Input: part model. Units: mm. Frame: model coordinates. Face numbers are marked on the shaded views. A direction names the side the tool comes from. Coordinates: 2 decimals unless noted, no trailing zeros. Write each loop counter-clockwise with the first axis right and the second up, starting at its lowest first coordinate (ties: lowest second). Pieces come first, ordered by that corner, then holes. Notation, with made-up numbers: (-4.5, 85.25) - (24.5, 85.25) arc R7 cw to (24.5, 98.25) - close; hole circle Ø6 at (87.5, 46). An arc over 180 degrees is marked (long way). Put each result on its own line as item: value. Start each with the question number.
1. Cut plane C-C, the plane y = 6.25. Return loops of the section in (x, z), and give its area (3 significant figures).
2. Cut plane D-D, the plane y = 2. Return loops of the section in (x, z).
3. Line query: line 1 (Z direction, x = 4, y = 5.5); line 2 (X direction, y = -0.2, z = -11.75); line 3 (Z direction, x = 18, y = -2). Output: solid intervals per line, ascending.
4. Pull-direction query (Z, two-part tool) for the marked faces 3, 4 and 5; classes: released by +Z, released by -Z, zero draft, split by the parting line, or undercut.
5. Cut plane B-B, the plane z = -11.75. Return loops of the section in (x, y), and give its area (3 significant figures).
6. Access query for the marked faces 1 and 2. Directions: +Z, -Z, +X, -X, +Y, -Y. A direction counts if a zero-diameter tool reaches every point of the face in a straight line with its end or side. Return the directions, or none.
7. Pin query (flat end, axial travel): pin 1 (11.5 mm diameter, centred on x = 17.5, z = 11.75, fed in from +Y); pin 2 (2.5 mm diameter, centred on y = -3.5, z = 15, fed in from -X); pin 3 (14.5 mm diameter, centred on x = 13, z = 1.5, fed in from +Y). Return the tip coordinate at first contact, or that it passes through.
8. Cut plane A-A, the plane x = 17.5. Return loops of the section in (y, z), and give its area (4 significant figures).
from build123d import *

# Parameters (mm, degrees)
EXTRUDE_1_DEPTH          = 22
PATTERN_LINEAR_1_COUNT   = 2
PATTERN_LINEAR_1_PITCH   = 23.5
CUT_EXTRUDE_1_DEPTH      = 38.269290307
CUT_EXTRUDE_1_DEPTH_BACK = 38.269290307
SKETCH_4_W               = 16.100903004
SKETCH_4_H               = 10.25
SKETCH_5_R               = 2.5
CUT_EXTRUDE_2_DEPTH      = 54.301031885


with BuildPart() as part:
    # 草图1 → 凸台-拉伸1 (new, symmetric)
    with BuildSketch(Plane.XY):
        with BuildLine():
            Line((29, -5.5), (29, -8))
            Line((29, -8), (1, -8))
            Line((1, -8), (-1.370141735, -7.373785434))
            ThreePointArc((-1.370141735, -7.373785434), (-4.794472702, 5.767411162), (7.5, 0))
            Line((7.5, 0), (25.406366901, 0))
            ThreePointArc((25.406366901, 0), (25.916831332, -0.140101131), (26.284262474, -0.521147869))
            Line((26.284262474, -0.521147869), (29, -5.5))
        make_face()
    extrude(amount=EXTRUDE_1_DEPTH, both=True)

    # 草图3 → 切除-旋转1 (revolve, cut)
    with BuildSketch(Plane.XY.offset(11.75), mode=Mode.PRIVATE) as cut_revolve_1_sk:
        Polygon((24, 0), (17.5, 0), (17.5, -8), (20.75, -8), (20.75, -4), (24, -1), align=None)
    cut_revolve_1 = revolve(cut_revolve_1_sk.sketch.rotate(Axis((17.5, -8, 11.75), (0, 1, 0)), 90), axis=Axis((17.5, -8, 11.75), (0, 1, 0)), mode=Mode.SUBTRACT)

    # 阵列(线性)1: 切除-旋转1 ×2
    with Locations(*[(0, 0, -i * PATTERN_LINEAR_1_PITCH) for i in range(1, PATTERN_LINEAR_1_COUNT)]):
        add(cut_revolve_1, mode=Mode.SUBTRACT)

    # 草图4 → 切除-拉伸1 (cut, two sides: drawn at the far end of the back side and taken through both)
    with BuildSketch(Plane(origin=(0, 0, 0), x_dir=(1, 0, 0), z_dir=(0, 1, 0)).offset(-CUT_EXTRUDE_1_DEPTH_BACK)):
        with Locations((-0.04685673, -16.875)):
            Rectangle(SKETCH_4_W, SKETCH_4_H)
        with Locations((-0.04685673, 5.625)):
            Rectangle(SKETCH_4_W, SKETCH_4_H)
    extrude(amount=CUT_EXTRUDE_1_DEPTH + CUT_EXTRUDE_1_DEPTH_BACK, mode=Mode.SUBTRACT)

    # 草图5 → 切除-拉伸2 (cut, through all)
    with BuildSketch(Plane(origin=(0, 0, -22), x_dir=(-1, 0, 0), z_dir=(0, 0, -1))):
        Circle(SKETCH_5_R)
    extrude(amount=-CUT_EXTRUDE_2_DEPTH, mode=Mode.SUBTRACT)


solid = part.part
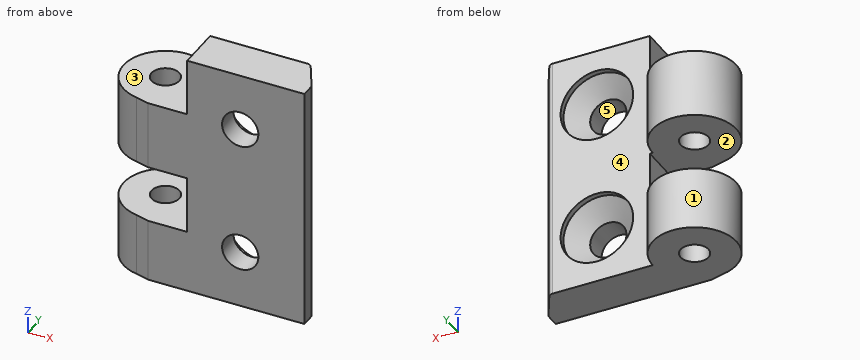
Report:
1. outline: (-4.15, -22) - (4.15, -22) - (4.15, -10.75) - (-4.15, -10.75) - close; (-4.15, -0.5) - (4.15, -0.5) - (4.15, 11.75) - (-4.15, 11.75) - close
1. area: 195 mm^2
2. outline: (-7.23, -22) - (-1.5, -22) - (-1.5, -10.75) - (-7.23, -10.75) - close; (-7.23, -0.5) - (-1.5, -0.5) - (-1.5, 11.75) - (-7.23, 11.75) - close; (1.5, -22) - (7.23, -22) - (7.23, -10.75) - (1.5, -10.75) - close; (1.5, -0.5) - (7.23, -0.5) - (7.23, 11.75) - (1.5, 11.75) - close
3. line 1: z = -22 to -10.75, -0.5 to 11.75
3. line 2: x = -7.5 to -2.49, 2.49 to 11, 24 to 26.01
3. line 3: z = -22 to -17.14, -6.36 to 6.36, 17.14 to 22
4. face 3: released by +Z
4. face 4: zero draft
4. face 5: undercut
5. outline: (-1.37, -7.37) - (1, -8) - (14.25, -8) - (14.25, -4) - (11, -1) - (11, 0) - (7.5, 0) arc R7.5 ccw (long way) to start; (20.75, -8) - (29, -8) - (29, -5.5) - (26.28, -0.52) arc R1 ccw to (25.41, 0) - (24, 0) - (24, -1) - (20.75, -4) - close; hole circle Ø5 at (0, 0)
5. area: 268 mm^2
6. face 1: +Z, -Z
6. face 2: -X, +Y, -Y
7. pin 1: stops at y = -1.69
7. pin 2: stops at x = 8
7. pin 3: stops at y = 4.82
8. outline: (-8, -22) - (0, -22) - (0, -18.25) - (-1, -18.25) - (-4, -15) - (-8, -15) - close; (-8, -8.5) - (-4, -8.5) - (-1, -5.25) - (0, -5.25) - (0, 5.25) - (-1, 5.25) - (-4, 8.5) - (-8, 8.5) - close; (-8, 15) - (-4, 15) - (-1, 18.25) - (0, 18.25) - (0, 22) - (-8, 22) - close
8. area: 215.5 mm^2
